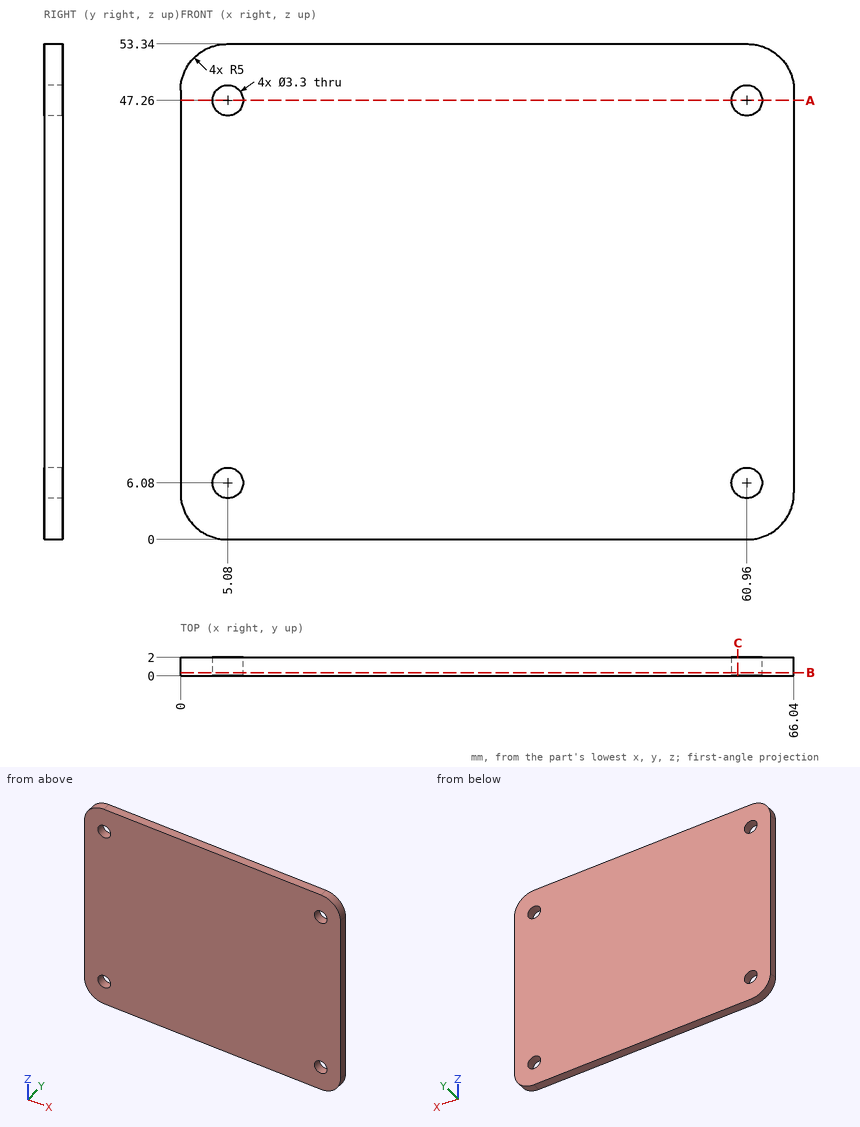
Geometry: see drawing. Coordinates: mm, zero at the bounding-box minimum. Round coordinates to 2 decimals unless told otherwise and drop trailing zeros. Order: outer loops, then holes, each group sorted by start corner. A loop starts at its lowest first (then second) coordinate and runs counter-clockwise, first axis right, second up. Notation, with made-up numbers: (82, 43) - (136, 43) arc R32 ccw to (136, 75) - close; hole circle Ø2 at (7, -12). An arc over 180 degrees is marked (long way). Use a Markdown table: item, result. Add a question column.
1. Line query: probe 1 along Z at (x, y) = (5.08, 1.45); probe 2 along X at (y, z) = (0.55, 46.5). Output: solid intervals per line, ascending.
2. Section query C-C (x = 60). Return the cut outline in (y, z).
3. Section query B-B (y = 0.35). Return the cut outline in (x, z).
4. Section query A-A (z = 47.26). Return the cut outline in (x, y), then the cut area to 3 significant figures.
5. First-contact query: pin 1 (2.5 mm diameter, centred on x = 5.08, z = 6.08, fed in from -Y). Flat tip, straight axial feed; report the tip coordinate or a pass-through.
Derived:
| question | item | result |
|---|---|---|
| 1 | probe 1 | 0 to 4.43, 7.73 to 45.61, 48.91 to 53.34 |
| 1 | probe 2 | 0 to 3.62, 6.54 to 59.5, 62.42 to 66.04 |
| 2 | outline | (0, 0) - (2, 0) - (2, 4.74) - (0, 4.74) - close; (0, 7.42) - (2, 7.42) - (2, 45.92) - (0, 45.92) - close; (0, 48.6) - (2, 48.6) - (2, 53.34) - (0, 53.34) - close |
| 3 | outline | (0, 5) arc R5 ccw to (5, 0) - (61.04, 0) arc R5 ccw to (66.04, 5) - (66.04, 48.34) arc R5 ccw to (61.04, 53.34) - (5, 53.34) arc R5 ccw to (0, 48.34) - close; hole circle Ø3.3 at (5.08, 6.08); hole circle Ø3.3 at (5.08, 47.26); hole circle Ø3.3 at (60.96, 6.08); hole circle Ø3.3 at (60.96, 47.26) |
| 4 | outline | (0, 0) - (3.43, 0) - (3.43, 2) - (0, 2) - close; (6.73, 0) - (59.31, 0) - (59.31, 2) - (6.73, 2) - close; (62.61, 0) - (66.04, 0) - (66.04, 2) - (62.61, 2) - close |
| 4 | area | 119 mm2 |
| 5 | pin 1 | through |
